Design review of the part built by this model. Coordinates are the model's own, in mm. Face numbers are marked on the shaded views. A direction names the side the tool comes from. Coordinates: 2 decimals unless noted, no trailing zeros. Loops run counter-clockwise (first coordinate to the right, second up) from the corner with the lowest first, then second, coordinate; pieces in that order, holes last. Notation, with made-up numbers: (4.25, 19) - (56.25, 19) arc R22 cw to (56.25, 57) - close; hole circle Ø7 at (0, -15). An arc over 180 degrees is marked (long way). One line per question, with ' | ' between items.
from build123d import *

# Parameters (mm, degrees)
SKETCH007_W     = 25.5
SKETCH007_H     = 62.15
PAD004_DEPTH    = 7.5
THICKNESS001_T  = 1.6
SKETCH008_R     = 9.6
POCKET002_DEPTH = 5
SKETCH009_W     = 27.1
SKETCH009_H     = 63.75
SKETCH009_W_2   = 25.5
SKETCH009_H_2   = 62.15
POCKET003_DEPTH = 0.8
FILLET001_R     = 0.8
SKETCH010_R     = 2.7
PAD005_DEPTH    = 7.5
SKETCH011_R     = 1.65
POCKET004_DEPTH = 3
SKETCH012_W     = 9.44
SKETCH012_H     = 3.495
POCKET005_DEPTH = 5


with BuildPart() as part:
    # Sketch007 (on Face1 of Binder001) → Pad004 (new body)
    with BuildSketch(Plane.XY.offset(1.51)):
        with Locations((12.5, 27.925)):
            Rectangle(SKETCH007_W, SKETCH007_H)
    extrude(amount=PAD004_DEPTH)

    # Thickness001
    thickness001_openings = [part.faces().sort_by_distance(p)[0] for p in [
        (12.5, 27.925, 1.51),
    ]]
    offset(amount=THICKNESS001_T, openings=thickness001_openings, kind=Kind.INTERSECTION)

    # Sketch008 (on Face11 of Thickness001) → Pocket002 (cut)
    with BuildSketch(Plane.XY.offset(10.61)):
        with Locations((12.5, 26)):
            Circle(SKETCH008_R)
    extrude(amount=-POCKET002_DEPTH, mode=Mode.SUBTRACT)

    # Sketch009 (on Face4 of Pocket002) → Pocket003 (cut)
    with BuildSketch(Plane(origin=(0, 0, 1.51), x_dir=(1, 0, 0), z_dir=(0, 0, -1))):
        with Locations((12.5, -27.925)):
            Rectangle(SKETCH009_W, SKETCH009_H)
        with Locations((12.5, -27.925)):
            Rectangle(SKETCH009_W_2, SKETCH009_H_2, mode=Mode.SUBTRACT)
    extrude(amount=-POCKET003_DEPTH, mode=Mode.SUBTRACT)

    # Fillet001
    fillet001_edges = [part.edges().sort_by_distance(p)[0] for p in [
        (26.85, -4.75, 6.06),
        (26.85, 60.6, 6.06),
        (-1.85, 60.6, 6.06),
        (-1.85, -4.75, 6.06),
    ]]
    fillet(fillet001_edges, radius=FILLET001_R)

    # Sketch010 (on Face21 of Fillet001) → Pad005 (join)
    with BuildSketch(Plane(origin=(0, 0, 9.01), x_dir=(1, 0, 0), z_dir=(0, 0, -1))):
        with Locations((2.5, -0.5)):
            Circle(SKETCH010_R)
        with Locations((22.5, -0.5)):
            Circle(SKETCH010_R)
        with Locations((2.5, -50)):
            Circle(SKETCH010_R)
        with Locations((22.5, -50)):
            Circle(SKETCH010_R)
    extrude(amount=PAD005_DEPTH)

    # Sketch011 (on Face27 of Pad005) → Pocket004 (cut)
    with BuildSketch(Plane(origin=(0, 0, 1.51), x_dir=(1, 0, 0), z_dir=(0, 0, -1))):
        with Locations((2.5, -0.5)):
            Circle(SKETCH011_R)
        with Locations((22.5, -0.5)):
            Circle(SKETCH011_R)
        with Locations((2.5, -50)):
            Circle(SKETCH011_R)
        with Locations((22.5, -50)):
            Circle(SKETCH011_R)
    extrude(amount=-POCKET004_DEPTH, mode=Mode.SUBTRACT)

    # Sketch012 (on Face20 of Pocket004) → Pocket005 (cut)
    with BuildSketch(Plane(origin=(0, -3.15, 0), x_dir=(-1, 0, 0), z_dir=(0, 1, 0))):
        with Locations((-12.5, 3.2575)):
            Rectangle(SKETCH012_W, SKETCH012_H)
    extrude(amount=-POCKET005_DEPTH, mode=Mode.SUBTRACT)


solid = part.part
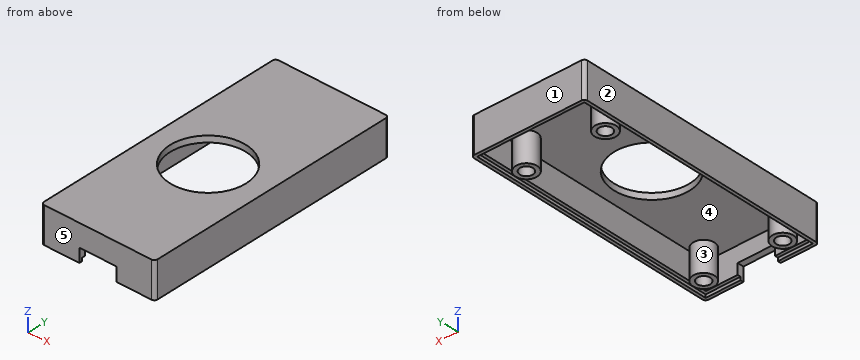
Q1. Take a section at A-A (x = 12.5). Give the boundary of the cut face in (y, z) (3 decimals), plus the area to 3 significant figures.
Returned:
outline: (-4.75, 5.005) - (-3.15, 5.005) - (-3.15, 9.01) - (16.4, 9.01) - (16.4, 10.61) - (-4.75, 10.61) - close; (35.6, 9.01) - (59, 9.01) - (59, 2.31) - (59.8, 2.31) - (59.8, 1.51) - (60.6, 1.51) - (60.6, 10.61) - (35.6, 10.61) - close | area: 91.6 mm²
Q2. To check wall thickness, follow line 1 along Y through (x, z) = (22.5, 4); line 2 along Y through (x, z) = (12.5, 9.95); line 3 along X through (y, z) = (8.5, 8). State the ranges of each line that lie inside material, in increasing order.
Returned:
line 1: y = -4.75 to -3.15, -2.2 to -1.15, 2.15 to 3.2, 47.3 to 48.35, 51.65 to 52.7, 59 to 60.6 | line 2: y = -4.75 to 16.4, 35.6 to 60.6 | line 3: x = -1.85 to -0.25, 25.25 to 26.85
Q3. For pin 1 (0.8 mm diameter, centred on x = 11.5, y = -4, fed in from -Z) (3 decimals); pin 2 (12 mm diameter, centred on x = 8.5, y = 25, fed in from +Z); pin 3 (1.6 mm diameter, centred on x = 22.5, y = 1, fed in from -Z); pin 4 (7.5 mm diameter, centred on x = 13.5, y = 20, fed in from -Z), all flat-tipped, find the tip position at first contact; note any pin that passes through.
Returned:
pin 1: stops at z = 5.005 | pin 2: stops at z = 10.61 | pin 3: stops at z = 4.51 | pin 4: stops at z = 9.01
Q4. Tool access review of the marked faces 4 and 5: name each direction out of +Z, -Z, +X, -X, +Y, -Y from which nothing blocks a thin tool from reaching the whole face with its end or side.
Returned:
face 4: -Z | face 5: +Z, -Z, +X, -X, -Y
Q5. Take a section at D-D (x = 23.25). Give the boundary of the cut face in (y, z), plus the area to 3 significant figures.
Returned:
outline: (-4.75, 1.51) - (-3.95, 1.51) - (-3.95, 2.31) - (-3.15, 2.31) - (-3.15, 9.01) - (-2.09, 9.01) - (-2.09, 1.51) - (-0.97, 1.51) - (-0.97, 4.51) - (1.97, 4.51) - (1.97, 1.51) - (3.09, 1.51) - (3.09, 9.01) - (47.41, 9.01) - (47.41, 1.51) - (48.53, 1.51) - (48.53, 4.51) - (51.47, 4.51) - (51.47, 1.51) - (52.59, 1.51) - (52.59, 9.01) - (59, 9.01) - (59, 2.31) - (59.8, 2.31) - (59.8, 1.51) - (60.6, 1.51) - (60.6, 10.61) - (-4.75, 10.61) - close | area: 187 mm²
Q6. Take a section at B-B (y = 26). Give the boundary of the cut face in (x, z).
Returned:
outline: (-1.85, 1.51) - (-1.05, 1.51) - (-1.05, 2.31) - (-0.25, 2.31) - (-0.25, 9.01) - (2.9, 9.01) - (2.9, 10.61) - (-1.85, 10.61) - close; (22.1, 9.01) - (25.25, 9.01) - (25.25, 2.31) - (26.05, 2.31) - (26.05, 1.51) - (26.85, 1.51) - (26.85, 10.61) - (22.1, 10.61) - close
Q7. Take a section at C-C (y = 44). Give the boundary of the cut face in (x, z), plus the area to 3 significant figures.
Returned:
outline: (-1.85, 1.51) - (-1.05, 1.51) - (-1.05, 2.31) - (-0.25, 2.31) - (-0.25, 9.01) - (25.25, 9.01) - (25.25, 2.31) - (26.05, 2.31) - (26.05, 1.51) - (26.85, 1.51) - (26.85, 10.61) - (-1.85, 10.61) - close | area: 68.6 mm²
Q8. Draft analysis for pull direction Y (two halves, no side actions). For the marked faces 1, 2 and 3, state which applies: +Y half, -Y half, draft (parallel to the pull), parting line (faces both ways), or undercut.
Returned:
face 1: +Y half | face 2: draft | face 3: undercut
